Could you check a few things on this model? Use its own coordinates, in mm. Give positions to 0.01 mm unless a question says otherwise; leave off trailing zeros. Order: outer loops, then holes, each group sorted by start corner. A loop starts at its lowest first (then second) coordinate and runs counter-clockwise, first axis right, second up. Notation, with made-up numbers: M 13.25,49 L 53.25,49 A23 ccw 53.25,76 Z; hole C 43.5,-35.5 d9. An arc over 180 degrees is marked long. Use a Markdown table: item, result. Add a question column.
Item 1: Suppose I cut it at B-B on x = -14.5. Write out the boundary of the cut face in (y, z).
Item 2: Suppose I cut it at A-A on z = 11. Write out the boundary of the cut face in (x, y), plus the area to 3 significant figures.
Item 3: Suppose I cut it at D-D on z = 36. Write out the boundary of the cut face in (x, y) (1 decimal), plus the area to 3 significant figures.
Item 4: I'm going to push flat-ended pins straight in: pin 1 Ø3 at (x, z) = (-13.49, 41.27) entering from +Y; pin 2 Ø2 at (x, z) = (-2.5, 39) entering from +Y; pin 3 Ø2 at (y, z) = (1.5, 9) entering from +X; pin 4 Ø6.5 at (x, z) = (-15.5, 31) entering from +Y. Where does each tip first touch, or does it pass through?
Item 5: Suppose I cut it at C-C on y = 4.5. Write out the boundary of the cut face in (x, z), plus the area to 3 significant figures.
Item 6: If I drill on L1, parallel to Z at x = -14, y = 1.25; L2, parallel to Y at x = -18, z = 47; L3, parallel to X at y = 1.25, z = 42, over which ranges is the centre line in solid material (lowest first)? Write a range as from..to.
from build123d import *

# Parameters (mm, degrees)
EXTRUDE1_DEPTH                      = 50.8
SKETCH2_W                           = 6.8326
SKETCH2_H                           = 25.4
CUT_EXTRUDE6_DEPTH                  = 56.557383842
EXTRUDE2_DEPTH                      = 50.8
SKETCH4_W                           = 6.8326
SKETCH4_H                           = 25.4
CUT_EXTRUDE7_DEPTH                  = 56.557383842
SKETCH5_R                           = 1.5875
EXTRUDE3_DEPTH                      = 25.4
SKETCH12_W                          = 2.413
SKETCH12_H                          = 1.8288
F_8_0_199_DIAMETER_HOLE1_AT_2_COUNT = 2
F_8_0_199_DIAMETER_HOLE1_AT_2_PITCH = 26.9875
F_8_0_199_DIAMETER_HOLE1_AT_3_COUNT = 2
F_8_0_199_DIAMETER_HOLE1_AT_3_PITCH = 41.669985076
F_8_0_199_DIAMETER_HOLE1_AT_4_COUNT = 2
F_8_0_199_DIAMETER_HOLE1_AT_4_PITCH = 31.75


with BuildPart() as part:
    # Sketch1 → Extrude1 (new body)
    with BuildSketch(Plane.XY):
        with BuildLine():
            Line((-21.43125, 0), (0, 0))
            ThreePointArc((0, 0), (1.779677423, 6.332436821), (-3.038247732, 1.8542))
            Line((-3.038247732, 1.8542), (-1.378132955, 2.628324234))
            ThreePointArc((-1.378132955, 2.628324234), (0.796631885, 4.789447439), (0, 1.8288))
            Line((0, 1.8288), (-21.43125, 1.8288))
            Line((-21.43125, 1.8288), (-21.43125, 0))
        make_face()
    extrude(amount=EXTRUDE1_DEPTH)

    # Sketch2 → Cut-Extrude6 (cut, through all)
    with BuildSketch(Plane(origin=(0, 0, 0), x_dir=(1, 0, 0), z_dir=(0, 1, 0))):
        with Locations((0, -12.7)):
            Rectangle(SKETCH2_W, SKETCH2_H)
    extrude(amount=CUT_EXTRUDE6_DEPTH, mode=Mode.SUBTRACT)


with BuildPart() as body_2:
    # Sketch3 → Extrude2 (new body)
    with BuildSketch(Plane.XY):
        with BuildLine():
            Line((0, 0), (21.43125, 0))
            Line((21.43125, 0), (21.43125, 1.8288))
            Line((21.43125, 1.8288), (3.025053626, 1.8288))
            ThreePointArc((3.025053626, 1.8288), (-1.767445818, 6.339866481), (0, 0))
        make_face()
    extrude(amount=EXTRUDE2_DEPTH)

    # Sketch4 → Cut-Extrude7 (cut, through all)
    with BuildSketch(Plane(origin=(0, 0, 0), x_dir=(1, 0, 0), z_dir=(0, 1, 0))):
        with Locations((0, -38.1)):
            Rectangle(SKETCH4_W, SKETCH4_H)
    extrude(amount=CUT_EXTRUDE7_DEPTH, mode=Mode.SUBTRACT)


with BuildPart() as body_3:
    # Sketch5 → Extrude3 (new body)
    with BuildSketch(Plane(origin=(0, 0, 25.4), x_dir=(-1, 0, 0), z_dir=(0, 0, -1))):
        with Locations((0, 3.4163)):
            Circle(SKETCH5_R)
    extrude(amount=-EXTRUDE3_DEPTH)

    # Sketch9 → Cut-Revolve1 (revolve, cut)
    with BuildSketch(Plane(origin=(0, 3.4163, 0), x_dir=(-1, 0, 0), z_dir=(0, 1, 0)), mode=Mode.PRIVATE) as cut_revolve1_sk:
        Polygon((-0.3175, 50.8), (-1.5875, 49.53), (-1.5875, 50.8), align=None)
    revolve(cut_revolve1_sk.sketch.rotate(Axis((0, 3.4163, 25.4), (0, 0, -1)), 180), axis=Axis((0, 3.4163, 25.4), (0, 0, -1)), mode=Mode.SUBTRACT)


with BuildPart() as body_2_1:
    add(body_2.part)

    # Combine1: union body 3
    add(body_3.part)

    # Sketch12 → #8 (0.199) Diameter Hole1 (revolve, cut)
    with BuildSketch(Plane(origin=(13.49375, 1.8288, 9.525), x_dir=(0, 0, 1), z_dir=(1, 0, 0))):
        with Locations((1.2065, 0.9144)):
            Rectangle(SKETCH12_W, SKETCH12_H)
    f_8_0_199_diameter_hole1 = revolve(axis=Axis((13.49375, 8.1788, 9.525), (0, -1, 0)), mode=Mode.SUBTRACT)

    # #8 (0.199) Diameter Hole1 at 4: #8 (0.199) Diameter Hole1 ×2
    with Locations(*[(0, 0, i * F_8_0_199_DIAMETER_HOLE1_AT_4_PITCH) for i in range(1, F_8_0_199_DIAMETER_HOLE1_AT_4_COUNT)]):
        add(f_8_0_199_diameter_hole1, mode=Mode.SUBTRACT)


with BuildPart() as part_1:
    add(part.part)

    # #8 (0.199) Diameter Hole1 at 2: #8 (0.199) Diameter Hole1 ×2
    with Locations(*[(-i * F_8_0_199_DIAMETER_HOLE1_AT_2_PITCH, 0, 0) for i in range(1, F_8_0_199_DIAMETER_HOLE1_AT_2_COUNT)]):
        add(f_8_0_199_diameter_hole1, mode=Mode.SUBTRACT)

    # #8 (0.199) Diameter Hole1 at 3: #8 (0.199) Diameter Hole1 ×2
    with Locations(*[Vector(-0.6476484200955402, 0, 0.7619393177594594) * (i * F_8_0_199_DIAMETER_HOLE1_AT_3_PITCH) for i in range(1, F_8_0_199_DIAMETER_HOLE1_AT_3_COUNT)]):
        add(f_8_0_199_diameter_hole1, mode=Mode.SUBTRACT)


solid = part_1.part
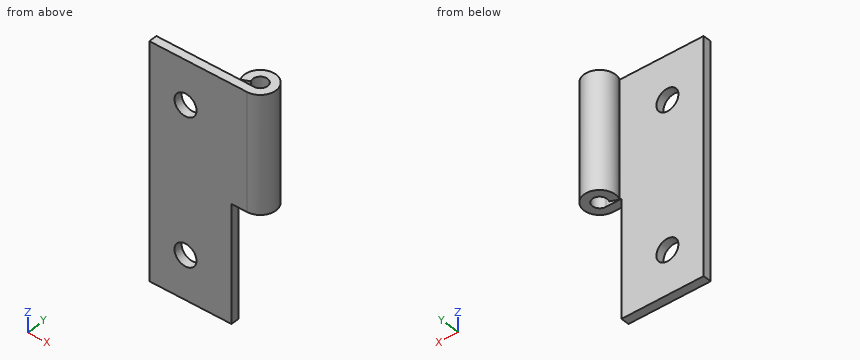
Findings below:
| question | item | result |
|---|---|---|
| 1 | outline | M 0,0 L 1.83,0 L 1.83,7.33 L 0,7.33 Z; M 0,11.72 L 1.83,11.72 L 1.83,39.08 L 0,39.08 Z; M 0,43.47 L 1.83,43.47 L 1.83,50.8 L 0,50.8 Z |
| 2 | outline | M -21.43,0 L -15.4,0 L -15.4,1.83 L -21.43,1.83 Z; M -11.58,0 L -3.42,0 L -3.42,1.83 L -11.58,1.83 Z |
| 2 | area | 26.0 mm^2 |
| 3 | outline | M -21.4,0 L 0,0 A3.4 ccw long -3,1.9 L -1.4,2.6 A1.6 cw long 0,1.8 L -21.4,1.8 Z |
| 3 | area | 63.0 mm^2 |
| 4 | pin 1 | passes through |
| 4 | pin 2 | stops at y = 6.49 |
| 4 | pin 3 | stops at x = -3.42 |
| 4 | pin 4 | stops at y = 1.83 |
| 5 | outline | M -3.24,25.4 L -1.16,25.4 L -1.16,50.8 L -3.24,50.8 Z; M 1.16,25.4 L 3.24,25.4 L 3.24,50.8 L 1.16,50.8 Z |
| 5 | area | 106 mm^2 |
| 6 | L1 | z = 0..7.17, 11.88..38.92, 43.63..50.8 |
| 6 | L2 | y = 0..1.83 |
| 6 | L3 | x = -21.43..-15.8, -11.19..2.64 |
